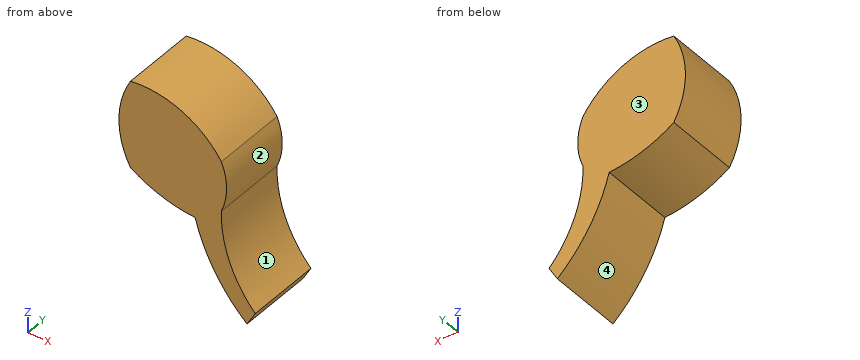
from build123d import *

# Parameters (mm, degrees)
F1_DEPTH = 12.7


with BuildPart() as f1:
    # F0 (on Front) → F1 (new body, symmetric)
    with BuildSketch(Plane.XZ):
        with BuildLine():
            ThreePointArc((29.999215, -30.187189), (31.719714, -22.004222), (29.999215, -13.821255))
            ThreePointArc((29.999215, -13.821255), (16.938376, -2.702505), (0, 0))
            ThreePointArc((0, 0), (-3.830529, -14.291319), (0, -28.582637))
            ThreePointArc((0, -28.582637), (10.192429, -33.65808), (21.339867, -35.977641))
            ThreePointArc((21.339867, -35.977641), (27.859584, -51.18178), (38.460912, -63.88156))
            Line((38.460912, -63.88156), (41.204112, -59.266559))
            ThreePointArc((41.204112, -59.266559), (32.703609, -45.843556), (29.999215, -30.187189))
        make_face()
    extrude(amount=F1_DEPTH, both=True)


solid = f1.part
Geometry check sheet. Reference: the model listing, model coordinates, mm. Face numbers are marked on the shaded views. Give positions to 0.01 mm unless a question says otherwise; leave off trailing zeros. Order: outer loops, then holes, each group sorted by start corner. A loop starts at its lowest first (then second) coordinate and runs counter-clockwise, first axis right, second up.
1. Sectioned sample at B-B (x = 12.5). Record the boundary of the cut face in (y, z), then the cut area to 3 significant figures.
Completed:
outline: (-12.7, -34.39) - (12.7, -34.39) - (12.7, -1.05) - (-12.7, -1.05) - close
area: 847 mm2
2. Draft check along Z on the marked faces 1, 2, 3 and 4. Enter one of: pulls with the +Z half, pulls with the -Z half, needs draft (parallel to the pull), parting line crosses it, or undercut.
Completed:
face 1: undercut
face 2: undercut
face 3: needs draft
face 4: pulls with the -Z half
3. Scan lines: line 1 (Z direction, x = 2.5, y = -6); line 2 (X direction, y = 7, z = -46.5); line 3 (X direction, y = 9.5, z = -41). Record each from-to range of solid material in increasing order.
Completed:
line 1: z = -30.14 to 0.19
line 2: x = 25.28 to 32.96
line 3: x = 22.93 to 31.18
4. Sectioned sample at C-C (z = -50). Record the boundary of the cut face in (x, y), then the cut area to 3 significant figures.
Completed:
outline: (27.15, -12.7) - (34.58, -12.7) - (34.58, 12.7) - (27.15, 12.7) - close
area: 189 mm2
5. Sectioned sample at A-A (y = 7.5). Record the boundary of the cut face in (x, z) (3 decimals), then the cut area to 3 significant figures.
Completed:
outline: (0, -28.583) arc R44.45 ccw to (21.34, -35.978) arc R57.15 ccw to (38.461, -63.882) - (41.204, -59.267) arc R40.64 cw to (29.999, -30.187) arc R20.32 ccw to (29.999, -13.821) arc R31.75 ccw to (0, 0) arc R28.575 ccw to start
area: 1,210 mm2
6. Depth check by flat-ended pin: pin 1 (10 mm diameter, centred on y = -4, z = -12, fed in from +X); pin 2 (2 mm diameter, centred on y = -3, z = -15, fed in from +X); pin 3 (10 mm diameter, centred on x = 24.5, y = -2, fed in from +Z). Enter the tip coordinate at first touch or a pass-through.
Completed:
pin 1: stops at x = 31.09
pin 2: stops at x = 30.81
pin 3: stops at z = -4.03
